```python
from build123d import *

# Parameters (mm, degrees)
SKETCH_W        = 75
SKETCH_H        = 55
PAD_DEPTH       = 3
SKETCH001_W     = 75
SKETCH001_H     = 55
SKETCH001_W_2   = 71
SKETCH001_H_2   = 51
PAD001_DEPTH    = 10
SKETCH002_W     = 5
SKETCH002_H     = 5
PAD002_DEPTH    = 5
SKETCH003_W     = 2
SKETCH003_H     = 19
POCKET_DEPTH    = 4
SKETCH004_W     = 2
SKETCH004_H     = 27
POCKET001_DEPTH = 4
SKETCH005_W     = 128
SKETCH005_H     = 15
PAD003_DEPTH    = 3
SKETCH006_R     = 2.5
POCKET002_DEPTH = 3
SKETCH007_W     = 16
SKETCH007_H     = 32
SKETCH007_R     = 3.25
SKETCH007_W_2   = 12
SKETCH007_H_2   = 15
PAD004_DEPTH    = 3
SKETCH010_W     = 7
SKETCH010_H     = 25
POCKET003_DEPTH = 3
SKETCH009_W     = 16
SKETCH009_H     = 19
SKETCH009_W_2   = 12
SKETCH009_H_2   = 15
PAD005_DEPTH    = 4
FILLET_R        = 10
FILLET001_R     = 3
FILLET002_R     = 3
FILLET003_R     = 3
FILLET004_R     = 3
FILLET005_R     = 7.5
FILLET006_R     = 7.49
FILLET007_R     = 7.49
FILLET008_R     = 7.5
SKETCH011_R     = 0.6
POCKET004_DEPTH = 5


with BuildPart() as part:
    # Sketch → Pad (new body)
    with BuildSketch(Plane.XY):
        with Locations((0, 27.5)):
            Rectangle(SKETCH_W, SKETCH_H)
    extrude(amount=PAD_DEPTH)

    # Sketch001 (on Face6 of Pad) → Pad001 (join)
    with BuildSketch(Plane.XY.offset(3)):
        with Locations((0, 27.5)):
            Rectangle(SKETCH001_W, SKETCH001_H)
        with Locations((0, 27.5)):
            Rectangle(SKETCH001_W_2, SKETCH001_H_2, mode=Mode.SUBTRACT)
    extrude(amount=PAD001_DEPTH)

    # Sketch002 (on Face15 of Pad001) → Pad002 (join)
    with BuildSketch(Plane.XY.offset(3)):
        with Locations((-33, 50.5)):
            Rectangle(SKETCH002_W, SKETCH002_H)
        with Locations((33, 50.5)):
            Rectangle(SKETCH002_W, SKETCH002_H)
        with Locations((33, 4.5)):
            Rectangle(SKETCH002_W, SKETCH002_H)
        with Locations((-33, 4.5)):
            Rectangle(SKETCH002_W, SKETCH002_H)
    extrude(amount=PAD002_DEPTH)

    # Sketch003 (on Face9 of Pad002) → Pocket (cut)
    with BuildSketch(Plane.XY.offset(13)):
        with Locations((36.5, 14.5)):
            Rectangle(SKETCH003_W, SKETCH003_H)
    extrude(amount=-POCKET_DEPTH, mode=Mode.SUBTRACT)

    # Sketch004 (on Face9 of Pocket) → Pocket001 (cut)
    with BuildSketch(Plane.XY.offset(13)):
        with Locations((-36.5, 20.5)):
            Rectangle(SKETCH004_W, SKETCH004_H)
    extrude(amount=-POCKET001_DEPTH, mode=Mode.SUBTRACT)

    # Sketch005 (on Face4 of Pocket001) → Pad003 (join)
    with BuildSketch(Plane(origin=(0, 0, 0), x_dir=(1, 0, 0), z_dir=(0, 0, -1))):
        with Locations((0, -7.5)):
            Rectangle(SKETCH005_W, SKETCH005_H)
    extrude(amount=-PAD003_DEPTH)

    # Sketch006 (on Face12 of Pad003) → Pocket002 (cut)
    with BuildSketch(Plane.XY.offset(3)):
        with Locations((-55, 7.5)):
            Circle(SKETCH006_R)
        with Locations((55, 7.5)):
            Circle(SKETCH006_R)
    extrude(amount=-POCKET002_DEPTH, mode=Mode.SUBTRACT)

    # Sketch007 (on Face4 of Pocket002) → Pad004 (join)
    with BuildSketch(Plane(origin=(0, 0, 0), x_dir=(1, 0, 0), z_dir=(0, 0, -1))):
        with Locations((-45.5, -31)):
            Rectangle(SKETCH007_W, SKETCH007_H)
        with Locations((-45.5, -40)):
            Circle(SKETCH007_R, mode=Mode.SUBTRACT)
        with Locations((-45.5, -23.5)):
            Rectangle(SKETCH007_W_2, SKETCH007_H_2, mode=Mode.SUBTRACT)
    extrude(amount=-PAD004_DEPTH)

    # Sketch010 (on Face46 of Pad004) → Pocket003 (cut)
    with BuildSketch(Plane.XY.offset(3)):
        with Locations((-32, 22.5)):
            Rectangle(SKETCH010_W, SKETCH010_H)
    extrude(amount=-POCKET003_DEPTH, mode=Mode.SUBTRACT)

    # Sketch009 (on Face22 of Pad004) → Pad005 (join)
    with BuildSketch(Plane.XY.offset(3)):
        with Locations((-45.5, 23.5)):
            Rectangle(SKETCH009_W, SKETCH009_H)
        with Locations((-45.5, 23.5)):
            Rectangle(SKETCH009_W_2, SKETCH009_H_2, mode=Mode.SUBTRACT)
    extrude(amount=PAD005_DEPTH)

    # Fillet
    fillet_edges = [part.edges().sort_by_distance(p)[0] for p in [
        (-53.5, 47, 1.5),
    ]]
    fillet(fillet_edges, radius=FILLET_R)

    # Fillet001
    fillet001_edges = [part.edges().sort_by_distance(p)[0] for p in [
        (37.5, 55, 8),
    ]]
    fillet(fillet001_edges, radius=FILLET001_R)

    # Fillet002
    fillet002_edges = [part.edges().sort_by_distance(p)[0] for p in [
        (-37.5, 55, 8),
    ]]
    fillet(fillet002_edges, radius=FILLET002_R)

    # Fillet003
    fillet003_edges = [part.edges().sort_by_distance(p)[0] for p in [
        (-37.5, 0, 8),
    ]]
    fillet(fillet003_edges, radius=FILLET003_R)

    # Fillet004
    fillet004_edges = [part.edges().sort_by_distance(p)[0] for p in [
        (37.5, 0, 8),
    ]]
    fillet(fillet004_edges, radius=FILLET004_R)

    # Fillet005
    fillet005_edges = [part.edges().sort_by_distance(p)[0] for p in [
        (64, 15, 1.5),
    ]]
    fillet(fillet005_edges, radius=FILLET005_R)

    # Fillet006
    fillet006_edges = [part.edges().sort_by_distance(p)[0] for p in [
        (64, 0, 1.5),
    ]]
    fillet(fillet006_edges, radius=FILLET006_R)

    # Fillet007
    fillet007_edges = [part.edges().sort_by_distance(p)[0] for p in [
        (-64, 0, 1.5),
    ]]
    fillet(fillet007_edges, radius=FILLET007_R)

    # Fillet008
    fillet008_edges = [part.edges().sort_by_distance(p)[0] for p in [
        (-64, 15, 1.5),
    ]]
    fillet(fillet008_edges, radius=FILLET008_R)

    # Sketch011 (on Face73 of Fillet008) → Pocket004 (cut)
    with BuildSketch(Plane.XY.offset(8)):
        with Locations((-33, 4.5)):
            Circle(SKETCH011_R)
        with Locations((33, 4.5)):
            Circle(SKETCH011_R)
        with Locations((-33, 50.5)):
            Circle(SKETCH011_R)
        with Locations((33, 50.5)):
            Circle(SKETCH011_R)
    extrude(amount=-POCKET004_DEPTH, mode=Mode.SUBTRACT)


solid = part.part
```
Build history of the part. All positions in model axes, mm. A direction names the side the tool comes from. Give positions to 0.01 mm unless a question says otherwise; leave off trailing zeros. Order: outer loops, then holes, each group sorted by start corner. A loop starts at its lowest first (then second) coordinate and runs counter-clockwise, first axis right, second up. Notation, with made-up numbers: M -4.75,42.5 L 53.25,42.5 A11 ccw 53.25,62.5 Z; hole C -19,51 d6. An arc over 180 degrees is marked long. Write item = value, one per line. Start each with the question number.
(1) Two-plate mould, pull along X, no slides. Class faces 1 (the flat face through (49, 7, 3)), 2 (the flat face through (33, 48, 5)), 3 (the cylindrical face through (-50.65, 43.99, 1.52)): released by +X, released by -X, zero draft, split by the parting line, or undercut.
(2) Pin check, flat tips, straight feed: pin 1 Ø15.5 at (x, y) = (17, 23) entering from +Z; pin 2 Ø1 at (x, z) = (-36.5, 12) entering from -Y; pin 3 Ø1.5 at (y, z) = (50, 6.5) entering from -X. Stop position of each tip, or through.
(3) Slice it at B-B on x = 9. Write the cut outline in (y, z).
(4) Which spindle directions (+Z, -Z, +X, -X, +Y, -Y) get a long thin tool onto all of the face, cutting with end or side? Do faces 4 (the flat face through (-46, 16, 3)), 5 (the cylindrical face through (36.6, 0.86, 8.07)), 6 (the cylindrical face through (-36.64, 0.9, 8.07)), 7 (the flat face through (32, 4, 8)), 8 (the flat face through (-55, 15, 1)). Say none if no direction does.
(5) Probe L1, parallel to Y at x = -33, z = 6.55; L2, parallel to X at y = 25, z = 4; L3, parallel to X at y = 50.5, z = 6.1. List the from-to ranges inside material, lowest first. Write a range as [from, to].
(6) Slice it at C-C on x = -45.5. Write the cut outline in (y, z), plus the area to 3 significant figures.
(7) Slice it at A-A on z = 5.5. State how many separate pieces and enclosed holes the cut face has, plus the area to 3 significant figures.
Responses:
q1.face_1 = zero draft
q1.face_2 = undercut
q1.face_3 = released by -X
q2.pin_1 = 3
q2.pin_2 = 0.4
q2.pin_3 = -37.5
q3.outline = M 0,0 L 55,0 L 55,13 L 53,13 L 53,3 L 2,3 L 2,13 L 0,13 Z
q4.face_4 = +Z, -Z
q4.face_5 = +Z, +X, -Y
q4.face_6 = +Z, -X, -Y
q4.face_7 = +Z
q4.face_8 = +Z, -Z, -X, +Y
q5.L1 = [0, 3.9], [5.1, 7], [48, 49.9], [51.1, 55]
q5.L2 = [-53.5, -51.5], [-39.5, -35.5], [35.5, 37.5]
q5.L3 = [-37.5, -33.6], [-32.4, -30.5], [30.5, 32.4], [33.6, 37.5]
q6.outline = M 0,0 L 16,0 L 16,7 L 14,7 L 14,3 L 0,3 Z; M 31,0 L 36.75,0 L 36.75,3 L 33,3 L 33,7 L 31,7 Z; M 43.25,0 L 46.8,0 L 46.8,3 L 43.25,3 Z
q6.area = 91.9 mm2
q7.separate_pieces = 1
q7.enclosed_holes = 6
q7.area = 716 mm2
